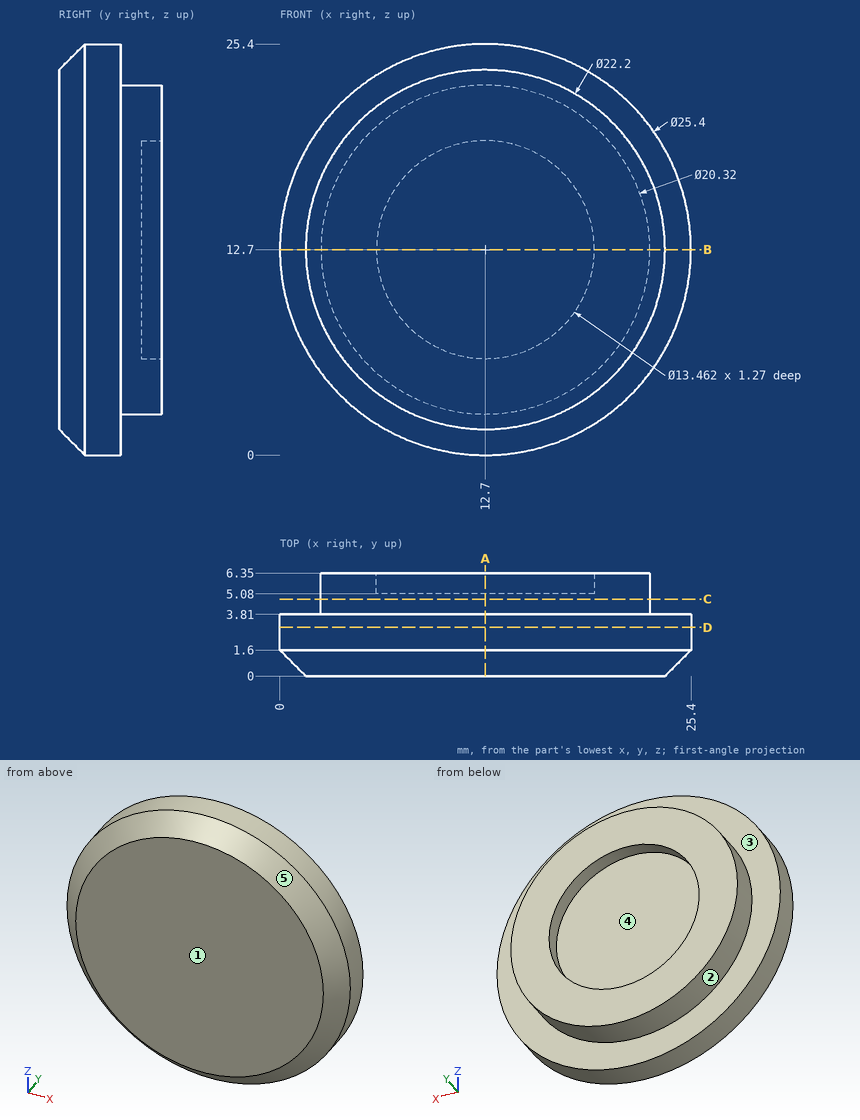
Could you check a few things on this drawing? It's one solid part, dimensions in mm from its lowest x, y, z. A direction names the side the tool comes from. Coordinates: 2 decimals unless noted, no trailing zeros. Order: outer loops, then holes, each group sorted by start corner. A loop starts at its lowest first (then second) coordinate and runs counter-clockwise, first axis right, second up.
1. For the marked faces 1 and 2, which set-ups out of +Z, -Z, +X, -X, +Y, -Y let a thin tool reach every point of the face, with its end or its side?
2. Thinking about a two-plate mould opening in Z: for the marked faces 3, 4 and 5, which applies, +Z half, -Z half, draft (parallel to the pull), parting line (faces both ways), or undercut?
3. If we section it at B-B (z = 12.7): Please give me the cut outline in (x, y), then the cut area to 3 significant figures.
4. If we section it at D-D (y = 3): Please give me the cut outline in (x, z), then the cut area to 3 significant figures.
5. I need wall thicknesses on line 1 (Z direction, x = 12.7, y = 6.1); line 2 (X direction, y = 1.75, z = 12.5); line 3 (Z direction, x = 14.75, y = 5.5). Which ranges of each line are inside material? Lowest first, please.
6. If we section it at C-C (y = 4.75): Please give me the cut outline in (x, z), then the cut area to 3 significant figures.
7. If we section it at A-A (x = 12.7): Please give me the cut outline in (y, z), then the cut area to 3 significant figures.
8. I'm going to push flat-ended pins straight in: pin 1 (1.5 mm diameter, centred on y = 0.5, z = 12, fed in from +X); pin 2 (1.5 mm diameter, centred on x = 14, z = 16, fed in from +Y); pin 3 (2 mm diameter, centred on y = 3.5, z = 7, fed in from +X). Where does each tip first touch, or does it pass through?
Entries:
1. face 1: +Z, -Z, +X, -X, -Y
1. face 2: +Y
2. face 3: draft
2. face 4: undercut
2. face 5: parting line
3. outline: (0, 1.6) - (1.6, 0) - (23.8, 0) - (25.4, 1.6) - (25.4, 3.81) - (22.86, 3.81) - (22.86, 6.35) - (19.43, 6.35) - (19.43, 5.08) - (5.97, 5.08) - (5.97, 6.35) - (2.54, 6.35) - (2.54, 3.81) - (0, 3.81) - close
3. area: 129 mm2
4. outline: circle Ø25.4 at (12.7, 12.7)
4. area: 507 mm2
5. line 1: z = 2.54 to 5.97, 19.43 to 22.86
5. line 2: x = 0 to 25.4
5. line 3: z = 2.75 to 6.29, 19.11 to 22.65
6. outline: circle Ø20.32 at (12.7, 12.7)
6. area: 324 mm2
7. outline: (0, 1.6) - (1.6, 0) - (3.81, 0) - (3.81, 2.54) - (6.35, 2.54) - (6.35, 5.97) - (5.08, 5.97) - (5.08, 19.43) - (6.35, 19.43) - (6.35, 22.86) - (3.81, 22.86) - (3.81, 25.4) - (1.6, 25.4) - (0, 23.8) - close
7. area: 129 mm2
8. pin 1: stops at x = 25.03
8. pin 2: stops at y = 5.08
8. pin 3: stops at x = 24.5
